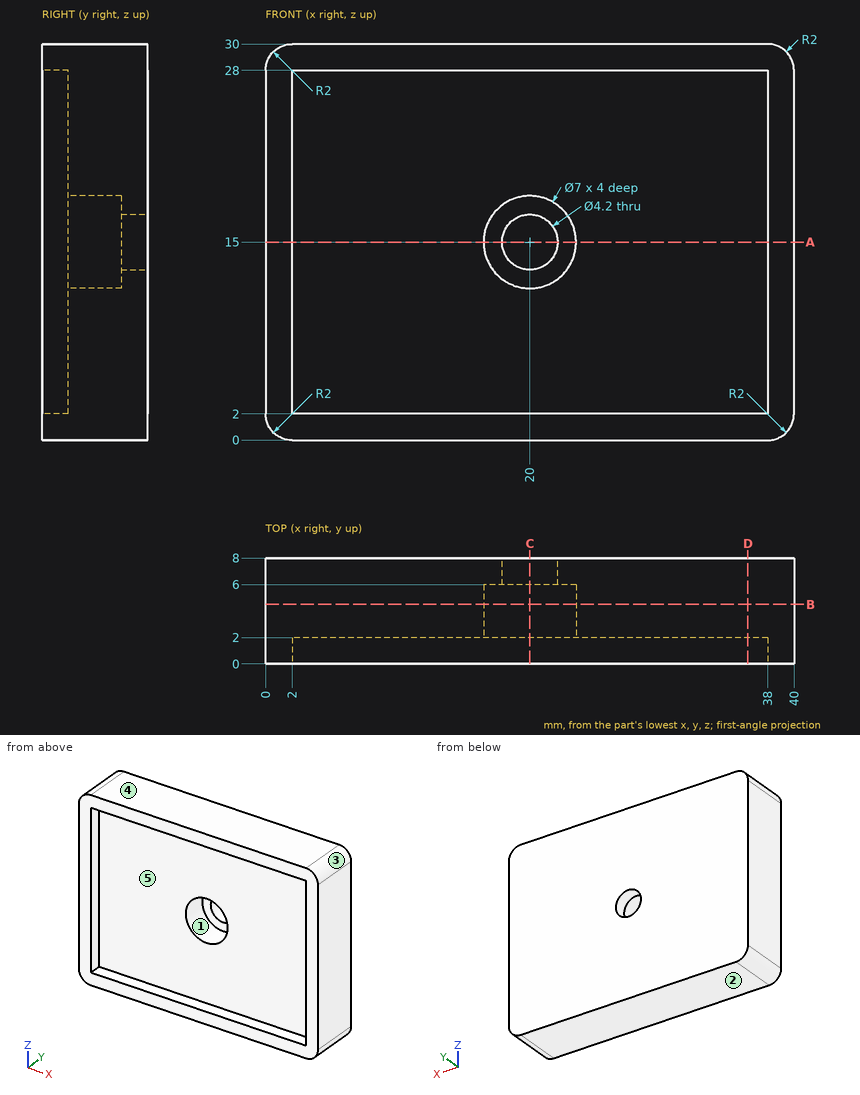
Verification items for this drawing (mm, ordinates from the low corner). A direction names the side the tool comes from. Coordinates: 2 decimals unless noted, no trailing zeros. Order: outer loops, then holes, each group sorted by start corner. A loop starts at its lowest first (then second) coordinate and runs counter-clockwise, first axis right, second up. Notation, with made-up numbers: (27.5, 7) - (70.5, 7) arc R25 cw to (70.5, 25) - close; hole circle Ø9 at (8, 61). An arc over 180 degrees is marked (long way). Answer in a Markdown table with one row per item. Add a question column.
1. Access from +Z, -Z, +X, -X, +Y, -Y to the whole of each face (thin tool, end or side, straight path). Record for the marked faces 1 and 2.
2. Section check D-D (x = 36.5). Enter the section's corners in (y, z), plus the area to 3 significant figures.
3. Section check C-C (x = 20). Enter the section's corners in (y, z), plus the area to 3 significant figures.
4. Section check B-B (y = 4.5). Enter the section's corners in (x, z), plus the area to 3 significant figures.
5. Material ranges on L1, parallel to X at y = 1.5, z = 4.75; L2, parallel to Z at x = 18.5, y = 1.5; L3, parallel to Z at x = 20, y = 7.2, recorded low to high. Write a range as [from, to].
6. Draft check along X on the marked faces 3, 4 and 5. Enter one of: +X half, -X half, draft (parallel to the pull), parting line (faces both ways), or undercut.
7. Section check A-A (z = 15). Enter the section's corners in (x, y).
8. Gauge pin test, flat end, axial feed: pin 1 Ø9 at (x, z) = (20, 15) entering from -Y. Record the tip position at first contact, or that the pin passes through.
Data:
| question | item | result |
|---|---|---|
| 1 | face 1 | -Y |
| 1 | face 2 | -Z, +X, -X, +Y, -Y |
| 2 | outline | (0, 0) - (8, 0) - (8, 30) - (0, 30) - (0, 28) - (2, 28) - (2, 2) - (0, 2) - close |
| 2 | area | 188 mm² |
| 3 | outline | (0, 0) - (8, 0) - (8, 12.9) - (6, 12.9) - (6, 11.5) - (2, 11.5) - (2, 2) - (0, 2) - close; (0, 28) - (2, 28) - (2, 18.5) - (6, 18.5) - (6, 17.1) - (8, 17.1) - (8, 30) - (0, 30) - close |
| 3 | area | 152 mm² |
| 4 | outline | (0, 2) arc R2 ccw to (2, 0) - (38, 0) arc R2 ccw to (40, 2) - (40, 28) arc R2 ccw to (38, 30) - (2, 30) arc R2 ccw to (0, 28) - close; hole circle Ø7 at (20, 15) |
| 4 | area | 1,160 mm² |
| 5 | L1 | x = [0, 2], [38, 40] |
| 5 | L2 | z = [0, 2], [28, 30] |
| 5 | L3 | z = [0, 12.9], [17.1, 30] |
| 6 | face 3 | +X half |
| 6 | face 4 | draft |
| 6 | face 5 | undercut |
| 7 | outline | (0, 0) - (2, 0) - (2, 2) - (16.5, 2) - (16.5, 6) - (17.9, 6) - (17.9, 8) - (0, 8) - close; (22.1, 6) - (23.5, 6) - (23.5, 2) - (38, 2) - (38, 0) - (40, 0) - (40, 8) - (22.1, 8) - close |
| 8 | pin 1 | stops at y = 2 |
